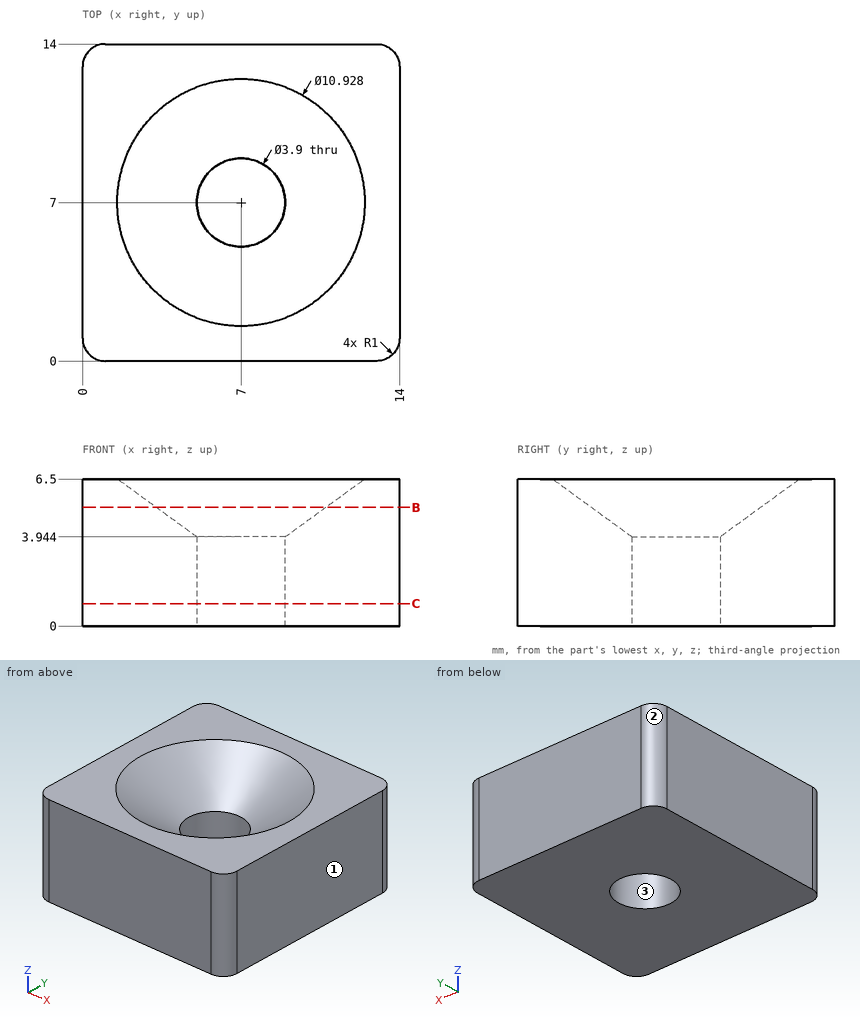
Part print with two shaded views. Sizes in mm from the minimum x, y, z corner. Round coordinates to 2 decimals unless told otherwise and drop trailing zeros. Order: outer loops, then holes, each group sorted by start corner. A loop starts at its lowest first (then second) coordinate and runs counter-clockwise, first axis right, second up.
(1) Drill centre lines: line 1 (X direction, y = 7, z = 1.95); line 2 (X direction, y = 8, z = 3.25) (1 decimal). Where is each one in solid material? Low to high.
(2) Pull direction Y, two halves, no side cores. Call the marked faces 1, 2 and 3: released by +Y, released by -Y, zero draft, split by the parting line, or undercut.
(3) Band-saw the part on B-B (z = 5.25). List the corners of the cut face in (x, y) (1 decimal).
(4) Band-saw the part on C-C (z = 1). List the corners of the cut face in (x, y).
(5) Pin check, flat tips, straight feed: pin 1 (1.5 mm diameter, centred on y = 4.5, z = 4, fed in from -X); pin 2 (2 mm diameter, centred on x = 4, y = 5.5, fed in from +Z); pin 3 (3 mm diameter, centred on x = 7, y = 7, fed in from +Z); pin 4 (1.5 mm diameter, centred on x = 9.5, y = 8.5, fed in from +Z). Stop position of each tip, or through.
Verdict:
1. line 1: x = 0 to 5.05, 8.95 to 14
1. line 2: x = 0 to 5.3, 8.7 to 14
2. face 1: zero draft
2. face 2: released by +Y
2. face 3: undercut
3. outline: (0, 1) arc R1 ccw to (1, 0) - (13, 0) arc R1 ccw to (14, 1) - (14, 13) arc R1 ccw to (13, 14) - (1, 14) arc R1 ccw to (0, 13) - close; hole circle Ø7.5 at (7, 7)
4. outline: (0, 1) arc R1 ccw to (1, 0) - (13, 0) arc R1 ccw to (14, 1) - (14, 13) arc R1 ccw to (13, 14) - (1, 14) arc R1 ccw to (0, 13) - close; hole circle Ø3.9 at (7, 7)
5. pin 1: stops at x = 0
5. pin 2: stops at z = 5.69
5. pin 3: passes through
5. pin 4: stops at z = 5.19
